Source: CAD feature listing. Evaluate the final solid. Frame: model axes, mm. Coordinates: 2 decimals unless noted, no trailing zeros. Order: outer loops, then holes, each group sorted by start corner. A loop starts at its lowest first (then second) coordinate and runs counter-clockwise, first axis right, second up.
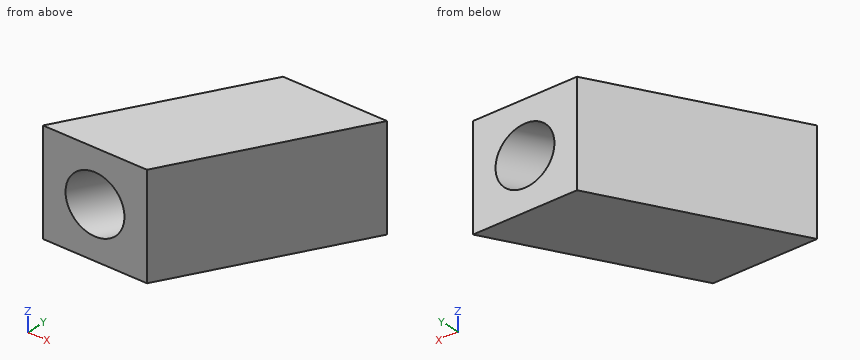
Autodesk Inventor part; units mm, degrees
ref_plane "YZ Plane" through (0, 0, 0) normal (1, 0, 0) x (0, 1, 0)
ref_plane "XZ Plane" through (0, 0, 0) normal (0, 1, 0) x (-1, 0, 0)
ref_plane "XY Plane" through (0, 0, 0) normal (0, 0, 1) x (1, 0, 0)
sketch "Sketch1" plane through (0, 0, 0) normal (0, 1, 0) x (-1, 0, 0)
  line L0 (0, 0) -> (15, 0)
  line L1 (15, 0) -> (15, -15)
  line L2 (15, -15) -> (0, -15)
  line L3 (0, -15) -> (0, 0)
  circle A0 centre (7.5, -7.5) radius 4.25
  dimension "soporte_largo" = 15
  dimension "soporte_ancho" = 15
  dimension "soporte_hueco_diametro" = 8.5
  dimension "soporte_hueco_pos_ancho" = 7.5
  dimension "soporte_hueco_pos_largo" = 7.5
sketch "Sketch2" plane through (0, 0, 0) normal (0, 0, 1) x (1, 0, 0)
  line L0 (0, 0) -> (14.4338, 25)
  line L1 (0, 0) -> (28.8675, 0) construction
  dimension "soporte_inclinacion" = 60
  dimension "soporte_alterura" = 25
sweep "Sweep1" add profiles "Sketch1" path "Sketch2"
equation "\"soporte_hueco_pos_ancho\" = 0.5 * soporte_ancho"
equation "\"soporte_hueco_pos_largo\" = 0.5 * soporte_largo"
equation "\"tol1\" = 0.1"
equation "\"tol2\" = 0.2"
equation "\"tol3\" = 0.3"
equation "\"tol4\" = 0.4"
equation "\"tol5\" = 0.5"
equation "\"tol6\" = 0.6"
equation "\"tol7\" = 0.7"
equation "\"tol8\" = 0.8"
equation "\"tol9\" = 0.9"
equation "\"tol\" = 7"
properties part number "TestSoporte"
Q1. Material intervals for line 1 along Z through (x, y) = (4.5, 21.25); line 2 along Z through (x, y) = (1.25, 13.5); line 3 along X through (y, z) = (5, -3.75), sorted ascending.
Solutions:
line 1: z = -15 to -11.74, -3.26 to 0
line 2: z = -15 to -11.64, -3.36 to 0
line 3: x = -12.11 to -6.61, -2.61 to 2.89
Q2. Pin query (flat end, axial travel): P1, Ø3, axis at y = 20.5, z = -8.5, coming from the +X side; P2, Ø8, axis at x = -11, z = -7, coming from the +Y side; P3, Ø3, axis at y = 14.5, z = -12.5, coming from the +X side. Return the tip coordinate at first contact, or that it passes through.
Solutions:
P1: stops at x = 12.7
P2: stops at y = 13.86
P3: stops at x = 9.24
Q3. Section query A-A on z = -13.75. Output: boundary loops of the cut face in (x, y), plus the area to 3 significant figures.
Solutions:
outline: (-15, 0) - (0, 0) - (14.43, 25) - (-0.57, 25) - close
area: 375 mm2
